Check sheet for the drawn part. Datum: minimum x, y, z corner. Units: mm. A direction names the side the tool comes from. Give positions to 0.01 mm unless a question says otherwise; leave off trailing zeros. Write each loop counter-clockwise with the first axis right and the second up, starting at its lowest first coordinate (ties: lowest second). Pieces come first, ordered by that corner, then holes. Notation, with made-up numbers: (-23, 49) -> (-18, 49) arc R31 cw to (-18, 81) -> close; hole circle Ø11 at (67, 17). An arc over 180 degrees is marked (long way). Use CSV: the item, a comma, the result in double quotes. Start each with the question number.
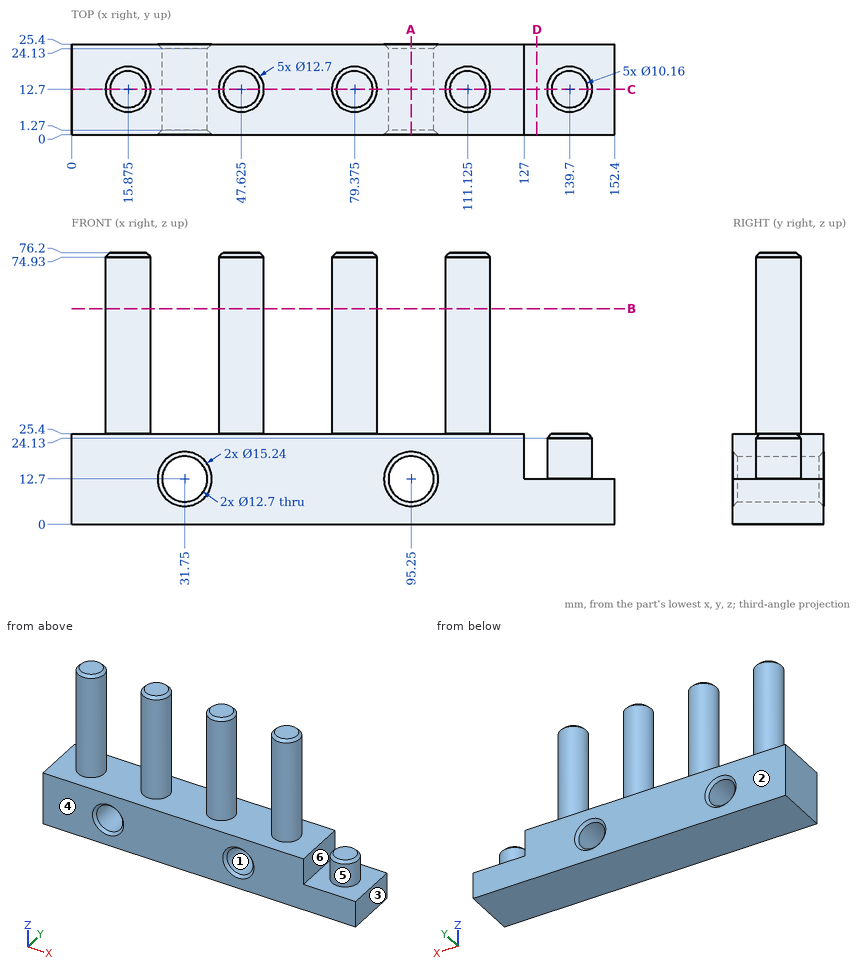
(1) Section check D-D on x = 130.5. Record the cut outline in (y, z), then the cut area to 3 significant figures.
(2) Section check B-B on z = 60.5. Record the cut outline in (x, y) (3 decimals), then the cut area to 3 significant figures.
(3) Go/stop test with flat-tipped pins: pin 1 (7.5 mm diameter, centred on x = 141.5, y = 6.5, fed in from +Z); pin 2 (10 mm diameter, centred on x = 108.5, z = 40, fed in from +Y); pin 3 (14.5 mm diameter, centred on x = 31.75, z = 12.7, fed in from +Y). Record where each tip stops, or that it passes through.
(4) Draft check along X on the marked faces 1, 2 and 3. Enter one of: released by +X, released by -X, zero draft, split by the parting line, or undercut.
(5) Set-up check for the marked faces 4, 5 and 6: record each of +Z, -Z, +X, -X, +Y, -Y from which the full face is reachable in a straight line by a thin tool's end or side.
(6) Section check C-C on y = 12.7. Give the number of separate pieces and of enclosed holes in the cut face, then the cut area to 3 significant figures.
(7) Section check A-A on x = 95.25. Record the cut outline in (y, z).
(8) Thickness scan on line 1 (Z direction, x = 31.75, y = 16.25); line 2 (X direction, y = 8, z = 7.5); line 3 (X direction, y = 2.5, z = 11.5). Record the ranges inside material, lowest first. Write a range as from..to.
Data:
1,outline,"(0, 0) -> (25.4, 0) -> (25.4, 12.7) -> (0, 12.7) -> close"
1,area,"323 mm2"
2,outline,"circle Ø12.7 at (15.875, 12.7); circle Ø12.7 at (47.625, 12.7); circle Ø12.7 at (79.375, 12.7); circle Ø12.7 at (111.125, 12.7)"
2,area,"507 mm2"
3,pin 1,"stops at z = 25.4"
3,pin 2,"stops at y = 19.05"
3,pin 3,"stops at y = 25.03"
4,face 1,"undercut"
4,face 2,"zero draft"
4,face 3,"released by +X"
5,face 4,"+Z, -Z, +X, -X, -Y"
5,face 5,"+Z"
5,face 6,"+Z, +Y, -Y"
6,separate pieces,"1"
6,enclosed holes,"2"
6,area,"6,030 mm2"
7,outline,"(0, 0) -> (25.4, 0) -> (25.4, 5.08) -> (24.13, 6.35) -> (1.27, 6.35) -> (0, 5.08) -> close; (0, 20.32) -> (1.27, 19.05) -> (24.13, 19.05) -> (25.4, 20.32) -> (25.4, 25.4) -> (0, 25.4) -> close"
8,line 1,"z = 0..6.35, 19.05..25.4"
8,line 2,"x = 0..28.11, 35.39..91.61, 98.89..152.4"
8,line 3,"x = 0..25.51, 37.99..89.01, 101.49..152.4"
